Autodesk Inventor part; units mm, degrees
ref_plane "YZ Plane" through (0, 0, 0) normal (1, 0, 0) x (0, 1, 0)
ref_plane "XZ Plane" through (0, 0, 0) normal (0, 1, 0) x (-1, 0, 0)
ref_plane "XY Plane" through (0, 0, 0) normal (0, 0, 1) x (1, 0, 0)
sketch "Sketch7" plane through (0, 0, 0) normal (0, 0, 1) x (1, 0, 0)
  line L0 (15, -12.5) -> (-15, -12.5)
  line L1 (-15, -12.5) -> (-15, 12.5)
  line L2 (-15, 12.5) -> (15, 12.5)
  line L3 (15, 12.5) -> (15, -12.5)
  line L4 (15, -12.5) -> (-15, 12.5) construction
  line L5 (-15, -12.5) -> (15, 12.5) construction
  point P0 (0, 0)
  dimension "d26" = 30
  dimension "d27" = 25
extrude "Extrusion4" add sketch "Sketch7" along normal blind 22
sketch "Sketch8" plane through (0, 0, 0) normal (0, 0, -1) x (-1, 0, 0)
  line L0 (-27, 12.5) -> (27, 12.5)
  line L1 (27, 12.5) -> (27, 3.5)
  line L2 (27, 3.5) -> (-27, 3.5)
  line L3 (-27, 3.5) -> (-27, 12.5)
  line L4 (-15, -12.5) -> (-15, 12.5)
  line L5 (15, 12.5) -> (15, -12.5)
  line L6 (-15, 12.5) -> (15, 12.5)
  point P0 (0, 0)
  dimension "d30" = 12
  dimension "d31" = 12
  dimension "d32" = 9
extrude "Extrusion5" add sketch "Sketch8" along normal blind 20
sketch "Sketch9" plane through (0, 0, 22) normal (0, 0, 1) x (1, 0, 0)
  line L0 (15, 12.5) -> (-15, 12.5)
  line L1 (15, -12.5) -> (15, 12.5)
  point P0 (0, 0)
  point P1 (0, 0)
  point P2 (0, 12.5)
  point P3 (15, 0)
hole "Hole3" at (0, 0, 22) direction (0, 0, -1) diameter 18.1 end through all
sketch "Sketch10" plane through (15, 3.5, 0) normal (0, -1, 0) x (1, 0, 0)
  line L0 (12, 0) -> (0, 0)
  line L1 (12, -20) -> (-6.6542, -20)
  line L2 (12, 0) -> (12, -20)
  line L3 (-42, 0) -> (-42, -20)
  point P0 (-15, 0)
  point P1 (4.5, -10)
  point P2 (-34.5, -10)
  dimension "d42" = 20
  dimension "d43" = 10
  dimension "d44" = 7.5
  dimension "d45" = 7.5
hole "Hole4" at (19.5, 3.5, -10) at (-19.5, 3.5, -10) direction (0, 1, 0) diameter 5.5 end through all
chamfer "Chamfer1" distance 2 angle 45 8 edges at (15, 12.5, 11) (15, -12.5, 11) (-15, -12.5, 11) (-15, 12.5, 11) (27, 8, 0) (27, 8, -20) (-27, 8, -20) (-27, 8, 0)
sketch "Sketch11" plane through (15, -10.5, 0) normal (1, 0, 0) x (0, 0, -1)
  line L0 (-22, 0) -> (-22, 21)
  point P0 (0, 10.5)
  point P1 (-14, 10.5)
  dimension "d63" = 8
hole "Hole5" at (15, 0, 14) direction (-1, 0, 0) diameter 4.134 end through all
equation "\"d31\" = d30"
properties part number "TL20240901-10320CV-026" material "MC NYLON"
Build history of the part. All positions in model axes, mm. A direction names the side the tool comes from. Coordinates: 2 decimals unless noted, no trailing zeros. Order: outer loops, then holes, each group sorted by start corner. A loop starts at its lowest first (then second) coordinate and runs counter-clockwise, first axis right, second up.
Item 1: Drop flat-ended pins along their axis: pin 1 Ø12 at (x, z) = (11, -15.5) entering from -Y; pin 2 Ø11 at (x, y) = (0, 0) entering from +Z; pin 3 Ø12 at (y, z) = (2.5, 8.5) entering from -X; pin 4 Ø2.5 at (x, y) = (-19, 9.5) entering from +Z. Give the stop position or say it passes through.
Filled in:
pin 1: stops at y = 3.5
pin 2: passes through
pin 3: stops at x = -15
pin 4: stops at z = 0
Item 2: Saw through at C-C on y = 0. List the corners of the cut face in (x, z), then the cut area to 3 significant figures.
Filled in:
outline: (-15, 0) - (-9.05, 0) - (-9.05, 11.93) - (-15, 11.93) - close; (-15, 16.07) - (-9.05, 16.07) - (-9.05, 22) - (-15, 22) - close; (9.05, 0) - (15, 0) - (15, 11.93) - (9.05, 11.93) - close; (9.05, 16.07) - (15, 16.07) - (15, 22) - (9.05, 22) - close
area: 213 mm2
Item 3: Saw through at D-D on z = 14. List the corners of the cut face in (x, y), then the cut area to 3 significant figures.
Filled in:
outline: (-15, -10.5) - (-13, -12.5) - (13, -12.5) - (15, -10.5) - (15, -2.07) - (8.81, -2.07) arc R9.05 cw to (-8.81, -2.07) - (-15, -2.07) - close; (-15, 2.07) - (-8.81, 2.07) arc R9.05 cw to (8.81, 2.07) - (15, 2.07) - (15, 10.5) - (13, 12.5) - (-13, 12.5) - (-15, 10.5) - close
area: 435 mm2
Item 4: Mould opens along Y. For faces 5 (the flat face through (-14, 11.5, 10.8)), 6 (the flat face through (26, 8, -1)), 7 (the cylindrical face through (-11.95, 0.79, 12.09)) say: released by +Y, released by -Y, zero draft, split by the parting line, or undercut.
Filled in:
face 5: released by +Y
face 6: zero draft
face 7: undercut
Item 5: Tool access for faces 1 (the flat face through (15, 0, 11)), 2 (the flat face through (-15, 0, 11)), 3 (the flat face through (0, -10, 0)), 4 (the flat face through (14, 11.5, 11.2)): list every direction of +Z, -Z, +X, -X, +Y, -Y with a clear straight run to the whole face (end or side of a thin tool).
Filled in:
face 1: +Z, +X, +Y, -Y
face 2: +Z, -X, +Y, -Y
face 3: -Z, +X, -X, -Y
face 4: +Z, +X, +Y
Item 6: Drill centre lines: L1, parallel to X at y = 10.25, z = -10; L2, parallel to X at y = -0.25, z = 17.5; L3, parallel to X at y = -2, z = 10.5. Where is each one in solid material? Low to high.
Filled in:
L1: x = -27 to -22.25, -16.75 to 16.75, 22.25 to 27
L2: x = -15 to -9.05, 9.05 to 15
L3: x = -15 to -8.83, 8.83 to 15
Item 7: Saw through at B-B on z = -10. List the corners of the cut face in (x, y), then the cut area to 3 significant figures.
Filled in:
outline: (-27, 3.5) - (-22.25, 3.5) - (-22.25, 12.5) - (-27, 12.5) - close; (-16.75, 3.5) - (-8.35, 3.5) arc R9.05 cw to (8.35, 3.5) - (16.75, 3.5) - (16.75, 12.5) - (-16.75, 12.5) - close; (22.25, 3.5) - (27, 3.5) - (27, 12.5) - (22.25, 12.5) - close
area: 320 mm2
Item 8: Saw through at A-A on x = 0. List the corners of the cut face in (y, z).
Filled in:
outline: (-12.5, 0) - (-9.05, 0) - (-9.05, 22) - (-12.5, 22) - close; (9.05, -20) - (12.5, -20) - (12.5, 22) - (9.05, 22) - close
